```python
from build123d import *

# Parameters (mm, degrees)
SKETCH1_W                  = 43.18
SKETCH1_H                  = 203.2
BOSS_EXTRUDE1_DEPTH        = 50.8
F_3_8_16_TAPPED_HOLE1_D    = 7.9375
F_10_32_TAPPED_HOLE1_D     = 4.0386
SKETCH9_W                  = 33.3375
SKETCH9_H                  = 50.596782444
CUT_EXTRUDE1_DEPTH         = 214.858346575
F_10_32_TAPPED_HOLE2_D     = 4.0386
F_10_32_TAPPED_HOLE2_DEPTH = 17.78
F_10_32_TAPPED_HOLE2_TIP   = 1.213317848
F_10_32_TAPPED_HOLE3_D     = 4.0386
F_10_32_TAPPED_HOLE3_DEPTH = 17.78
F_10_32_TAPPED_HOLE3_TIP   = 1.213317848


with BuildPart() as part:
    # Sketch1 → Boss-Extrude1 (new body)
    with BuildSketch(Plane.XY):
        with Locations((-21.59, 23.319966314)):
            Rectangle(SKETCH1_W, SKETCH1_H)
    extrude(amount=BOSS_EXTRUDE1_DEPTH)

    # 3/8-16 Tapped Hole1 (through all)
    with Locations(Plane.XY.offset(50.8)):
        with Locations((-21.59, 108.409966314), (-21.59, -61.770033686)):
            Hole(F_3_8_16_TAPPED_HOLE1_D / 2)

    # #10-32 Tapped Hole1 (through all)
    with Locations(Plane(origin=(0, 0, 0), x_dir=(0, 0, -1), z_dir=(1, 0, 0))):
        with Locations((-36.5125, 99.519966314), (-36.5125, 23.319966314), (-36.5125, -52.880033686)):
            Hole(F_10_32_TAPPED_HOLE1_D / 2)

    # Sketch9 → Cut-Extrude1 (cut, through all)
    with BuildSketch(Plane(origin=(0, 124.919966314, 0), x_dir=(1, 0, 0), z_dir=(0, 1, 0))):
        with Locations((-21.81225, -17.564108778)):
            Rectangle(SKETCH9_W, SKETCH9_H)
    extrude(amount=-CUT_EXTRUDE1_DEPTH, mode=Mode.SUBTRACT)

    # #10-32 Tapped Hole2
    with Locations(Plane(origin=(3.175, 53.792091732, -9.087092082), x_dir=(0, 0, -1), z_dir=(1, 0, 0))):
        with Locations((284.600407918, 58.427874582), (310.000407918, 58.427874582), (284.600407918, 13.977874582), (310.000407918, 13.977874582), (284.600407918, -30.472125418), (284.600407918, -74.922125418), (310.000407918, -74.922125418), (284.600407918, -119.372125418), (310.000407918, -119.372125418), (-20.199592082, 58.427874582), (-45.599592082, 58.427874582), (-20.199592082, 13.977874582), (-45.599592082, 13.977874582), (-20.199592082, -30.472125418), (-20.199592082, -74.922125418), (-45.599592082, -74.922125418), (-45.599592082, -119.372125418), (-20.199592082, -119.372125418)):
            Hole(F_10_32_TAPPED_HOLE2_D / 2, depth=F_10_32_TAPPED_HOLE2_DEPTH)
            with Locations((0, 0, -(F_10_32_TAPPED_HOLE2_DEPTH + F_10_32_TAPPED_HOLE2_TIP / 2))):  # 118° drill point
                Cone(0, F_10_32_TAPPED_HOLE2_D / 2, F_10_32_TAPPED_HOLE2_TIP, mode=Mode.SUBTRACT)

    # #10-32 Tapped Hole3
    with Locations(Plane(origin=(3.175, -7.152159104, -273.487907918), x_dir=(0, 0, 1), z_dir=(1, 0, 0))):
        with Locations((284.600407918, 58.427874582), (310.000407918, 58.427874582), (284.600407918, 13.977874582), (310.000407918, 13.977874582), (284.600407918, -30.472125418), (284.600407918, -74.922125418), (310.000407918, -74.922125418), (284.600407918, -119.372125418), (310.000407918, -119.372125418), (-20.199592082, 58.427874582), (-45.599592082, 58.427874582), (-20.199592082, 13.977874582), (-45.599592082, 13.977874582), (-20.199592082, -30.472125418), (-20.199592082, -74.922125418), (-45.599592082, -74.922125418), (-45.599592082, -119.372125418), (-20.199592082, -119.372125418)):
            Hole(F_10_32_TAPPED_HOLE3_D / 2, depth=F_10_32_TAPPED_HOLE3_DEPTH)
            with Locations((0, 0, -(F_10_32_TAPPED_HOLE3_DEPTH + F_10_32_TAPPED_HOLE3_TIP / 2))):  # 118° drill point
                Cone(0, F_10_32_TAPPED_HOLE3_D / 2, F_10_32_TAPPED_HOLE3_TIP, mode=Mode.SUBTRACT)


solid = part.part
```
The listing builds one solid part. Answer for the finished solid, in the listing's coordinates (mm). A direction names the side the tool comes from. Give positions to 0.01 mm unless a question says otherwise; leave off trailing zeros. Order: outer loops, then holes, each group sorted by start corner. A loop starts at its lowest first (then second) coordinate and runs counter-clockwise, first axis right, second up. Notation, with made-up numbers: (55, 85.25) - (95, 85.25) arc R9 cw to (95, 98.25) - close; hole circle Ø3 at (-35, 70). An arc over 180 degrees is marked (long way). Answer in a Markdown table with one row per item. Add a question column.
Q1. The part is cut by section B-B (z = 19). Determine the outline of the cut face in (x, y).
Q2. The part is cut by section D-D (x = -32). Determine the outline of the cut face in (y, z), then the cut area to 3 significant figures.
Q3. Which of the six approach directions +Z, -Z, +X, -X, +Y, -Y give full straight-line access (tool end or side, diameter ignored) to faces 1 (the flat face through (0, 22, 25)), 2 (the cylindrical face through (-2.608, 114.222, 10.85)), 3 (the flat face through (-5.143, 25, 22))?
Q4. Given P1, Ø2.5, axis at y = -65.58, z = 36.51, coming from the +X side; P2, Ø10, axis at x = -26, y = 22.5, coming from the -Z side, each flat-ended and moving along its own axis, determine where each tip first touches the part or whether it passes through.
Q5. For a pull along Z with two mould halves and no side action, classify faces 4 (the flat face through (-22, 25, 50.8)), 5 (the cylindrical face through (-18.665, -59.088, 46.776)), 6 (the cylindrical face through (-2.608, 21.528, 37.444)), 7 (the cylindrical face through (-2.608, -19.128, 10.85)) as released by +Z, released by -Z, zero draft, split by the parting line, or undercut.
Q6. The part is cut by section C-C (y = 75). Determine the outline of the cut face in (x, z), then the cut area to 3 significant figures.
Q7. Find the intervals of material crossed by line 1 along Y through (x, z) = (-21.59, 45.5); line 2 along X through (y, z) = (115, 19.5); line 3 along Z through (x, y) = (-36.5, 106), in increasing order. Write a range as [from, to].
Q8. The part is cut by section A-A (x = -21.59). Determine the outline of the cut face in (y, z).
Determined:
| question | item | result |
|---|---|---|
| 1 | outline | (-43.18, -78.28) - (-38.48, -78.28) - (-38.48, 124.92) - (-43.18, 124.92) - close; (-5.14, -78.28) - (0, -78.28) - (0, 124.92) - (-5.14, 124.92) - close |
| 2 | outline | (-78.28, 42.86) - (124.92, 42.86) - (124.92, 50.8) - (-78.28, 50.8) - close |
| 2 | area | 1,610 mm² |
| 3 | face 1 | +Z, -Z, +X, +Y, -Y |
| 3 | face 2 | +X |
| 3 | face 3 | -Z, +Y, -Y |
| 4 | P1 | stops at x = -38.48 |
| 4 | P2 | stops at z = 42.86 |
| 5 | face 4 | released by +Z |
| 5 | face 5 | zero draft |
| 5 | face 6 | undercut |
| 5 | face 7 | undercut |
| 6 | outline | (-43.18, 0) - (-38.48, 0) - (-38.48, 42.86) - (-5.14, 42.86) - (-5.14, 0) - (0, 0) - (0, 50.8) - (-43.18, 50.8) - close |
| 6 | area | 765 mm² |
| 7 | line 1 | y = [-78.28, -65.74], [-57.8, 104.44], [112.38, 124.92] |
| 7 | line 2 | x = [-43.18, -38.48], [-5.14, 0] |
| 7 | line 3 | z = [42.86, 50.8] |
| 8 | outline | (-78.28, 42.86) - (-65.74, 42.86) - (-65.74, 50.8) - (-78.28, 50.8) - close; (-57.8, 42.86) - (104.44, 42.86) - (104.44, 50.8) - (-57.8, 50.8) - close; (112.38, 42.86) - (124.92, 42.86) - (124.92, 50.8) - (112.38, 50.8) - close |
